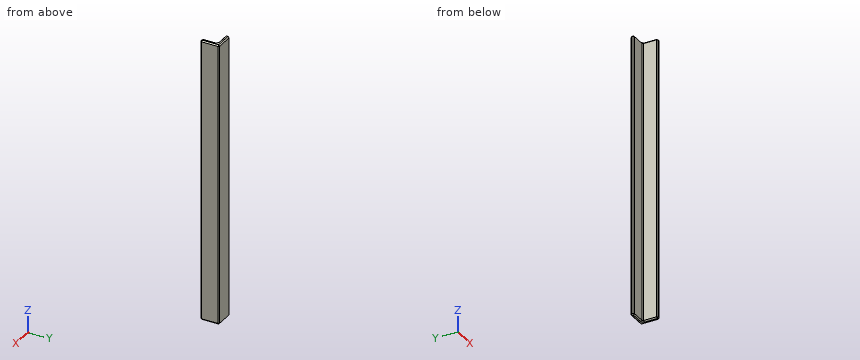
from build123d import *

# Parameters (mm, degrees)
BOX001_W     = 40
BOX001_H     = 40
BOX001_DEPTH = 750
BOX_W        = 50
BOX_H        = 50
BOX_DEPTH    = 750
CHAMFER_SIZE = 3


with BuildPart() as cube001:
    # Box001 → Box001 (new body)
    with BuildSketch(Plane.XY):
        with Locations((20, 20)):
            Rectangle(BOX001_W, BOX001_H)
    extrude(amount=BOX001_DEPTH)


with BuildPart() as chamfer_body:
    # Box → Box (new body)
    with BuildSketch(Plane.XY):
        with Locations((25, 25)):
            Rectangle(BOX_W, BOX_H)
    extrude(amount=BOX_DEPTH)

    # Cut: cut Cube001
    add(cube001.part, mode=Mode.SUBTRACT)

    # Chamfer
    chamfer_edges = [chamfer_body.edges().sort_by_distance(p)[0] for p in [
        (0, 40, 375),
        (0, 45, 750),
        (0, 50, 375),
        (0, 45, 0),
        (20, 40, 0),
        (40, 40, 375),
        (20, 40, 750),
        (25, 50, 750),
        (50, 25, 750),
        (45, 0, 750),
        (40, 20, 750),
        (25, 50, 0),
        (50, 50, 375),
        (50, 25, 0),
        (45, 0, 0),
        (40, 20, 0),
        (40, 0, 375),
        (50, 0, 375),
    ]]
    chamfer(chamfer_edges, length=CHAMFER_SIZE)


solid = chamfer_body.part
Work out the finished part from the listing and answer in its coordinate system (mm). Give positions to 0.01 mm unless a question says otherwise; leave off trailing zeros. Loops run counter-clockwise (first coordinate to the right, second up) from the corner with the lowest first, then second, coordinate; pieces in that order, holes last. Notation, with made-up numbers: (-17, 5.5) -> (-12, 5.5) arc R22 cw to (-12, 34.5) -> close; hole circle Ø6 at (51.5, 73.25). An arc over 180 degrees is marked (long way). Use a Markdown table: item, result. Add a question column.
1) The part is cut by section A-A, the plane x = 29. Determine the outline of the cut face in (y, z).
2) Each of these flat-tipped pins is pushed along its axis until it touches: P1, Ø1.5, axis at x = 39.5, z = 313, coming from the -Y side; P2, Ø6, axis at y = 11, z = 557, coming from the -X side; P3, Ø6, axis at x = 13, z = 108.5, coming from the -Y side. Where does it stop, or does it pass through?
3) The part is cut by section B-B, the plane z = 98. Determine the outline of the cut face in (x, y), plus the area to 3 significant figures.
4) Consider line 1 along Y through (x, z) = (27.5, 645); line 2 along Z through (x, y) = (34, 47.5). Determine where each line is inside the solid, lowest interval first.
Reported:
| question | item | result |
|---|---|---|
| 1 | outline | (40, 3) -> (43, 0) -> (47, 0) -> (50, 3) -> (50, 747) -> (47, 750) -> (43, 750) -> (40, 747) -> close |
| 2 | P1 | stops at y = 2.75 |
| 2 | P2 | stops at x = 40 |
| 2 | P3 | stops at y = 40 |
| 3 | outline | (0, 43) -> (3, 40) -> (37, 40) -> (40, 37) -> (40, 3) -> (43, 0) -> (47, 0) -> (50, 3) -> (50, 47) -> (47, 50) -> (3, 50) -> (0, 47) -> close |
| 3 | area | 882 mm^2 |
| 4 | line 1 | y = 40 to 50 |
| 4 | line 2 | z = 0.5 to 749.5 |
